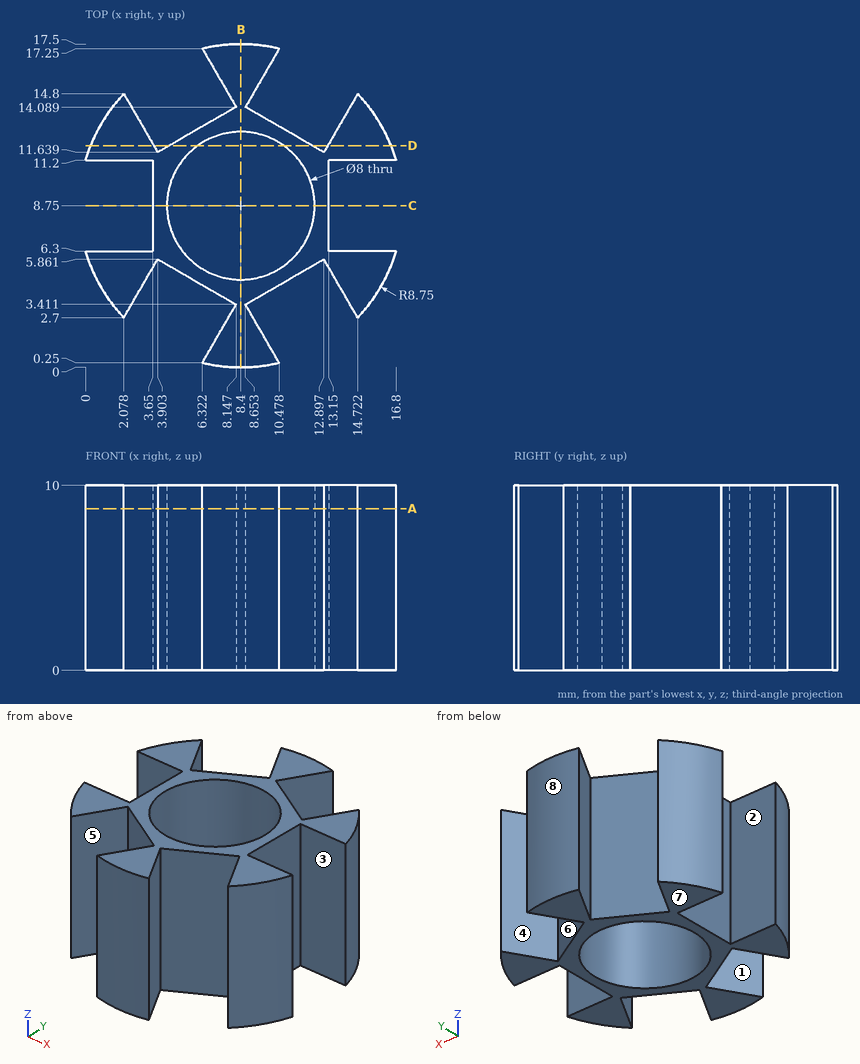
For this review, use the dimensioned drawing (mm, ordinates from the lowest corner) and the shaded views. A direction names the side the tool comes from. Coordinates: 2 decimals unless noted, no trailing zeros. Loops run counter-clockwise (first coordinate to the right, second up) from the corner with the lowest first, then second, coordinate; pieces in that order, holes last. Notation, with made-up numbers: M 33.25,64 L 81.25,64 A10 cw 81.25,70 Z; hole C 28.25,3.5 d1. An arc over 180 degrees is marked long. Answer as CSV lines item,"result".
Item 1: Machinability: for the marked faces 1, 2, 3, 4 and 5, which of the approach directions +Z, -Z, +X, -X, +Y, -Y give a long, thin tool a straight path to every point of the face, cutting with its end or side? Answer none if there is none.
Answer list:
face 1,"+Z, -Z"
face 2,"+Z, -Z, -X"
face 3,"+Z, -Z, +X"
face 4,"+Z, -Z, +Y"
face 5,"+Z, -Z, -Y"
Item 2: The part is to be moulded in two halves that separate along X. For the marked faces 6, 7 and 8, say which applies: pulls with the +X half, pulls with the -X half, needs draft (parallel to the pull), parting line crosses it, or undercut.
Answer list:
face 6,"undercut"
face 7,"needs draft"
face 8,"parting line crosses it"
Item 3: Add section D-D on y = 12. State the section outline as (x, z) points (1 decimal).
Answer list:
outline,"M 0.3,0 L 3.7,0 L 3.7,10 L 0.3,10 Z; M 4.5,0 L 6.1,0 L 6.1,10 L 4.5,10 Z; M 10.7,0 L 12.3,0 L 12.3,10 L 10.7,10 Z; M 13.1,0 L 16.5,0 L 16.5,10 L 13.1,10 Z"
Item 4: Add section A-A on z = 8.75. State the section outline as (x, y) points.
Answer list:
outline,"M 0,6.3 A8.75 ccw 2.08,2.7 L 3.9,5.86 L 8.15,3.41 L 6.32,0.25 A8.75 ccw 10.48,0.25 L 8.65,3.41 L 12.9,5.86 L 14.72,2.7 A8.75 ccw 16.8,6.3 L 13.15,6.3 L 13.15,11.2 L 16.8,11.2 A8.75 ccw 14.72,14.8 L 12.9,11.64 L 8.65,14.09 L 10.48,17.25 A8.75 ccw 6.32,17.25 L 8.15,14.09 L 3.9,11.64 L 2.08,14.8 A8.75 ccw 0,11.2 L 3.65,11.2 L 3.65,6.3 Z; hole C 8.4,8.75 d8"
Item 5: For P1, Ø4, axis at x = 16, z = 6.5, coming from the +Y side; P2, Ø9, axis at x = 8.4, y = 8.75, coming from the +Z side; P3, Ø1.5, axis at y = 9, z = 5.5, coming from the -X side; P4, Ø3, axis at x = 15, z = 6, coming from the -Y side, all flat-tipped, find the tip position at first contact; note any pin that passes through.
Answer list:
P1,"y = 14.8"
P2,"z = 10"
P3,"x = 3.65"
P4,"y = 2.7"
Item 6: For probe 1 along Y at (x, z) = (8, 6.25) (1 decimal); probe 2 along Y at (x, z) = (8.25, 5.5); probe 3 along X at (y, z) = (11, 1.5), list the stretches that pass through material, from the lowest coordinate up.
Answer list:
probe 1,"0 to 3.2, 3.5 to 4.8, 12.7 to 14, 14.3 to 17.5"
probe 2,"0 to 4.75, 12.75 to 17.5"
probe 3,"3.65 to 5.09, 11.71 to 13.15"
Item 7: Add section C-C on y = 8.75. State the section outline as (x, z) points.
Answer list:
outline,"M 3.65,0 L 4.4,0 L 4.4,10 L 3.65,10 Z; M 12.4,0 L 13.15,0 L 13.15,10 L 12.4,10 Z"
Item 8: Add section B-B on x = 8.4. State the section outline as (y, z) points.
Answer list:
outline,"M 0,0 L 4.75,0 L 4.75,10 L 0,10 Z; M 12.75,0 L 17.5,0 L 17.5,10 L 12.75,10 Z"
